Part model, mm, in its own coordinate system. Face numbers are marked on the shaded views. Give positions to 0.01 mm unless a question says otherwise; leave off trailing zeros. Loops run counter-clockwise (first coordinate to the right, second up) from the corner with the lowest first, then second, coordinate; pieces in that order, holes last. Notation, with made-up numbers: (53, 56) -> (85, 56) arc R15 ccw to (85, 60) -> close; hole circle Ø11 at (20, -1). An arc over 180 degrees is marked (long way). Write item = value, one per line.
from build123d import *

# Parameters (mm, degrees)
F3_R     = 3.8930000325
F4_DEPTH = 12.001


# Not quite as in the source:
# - a fillet or chamfer that OpenCascade refuses, or shapes differently, is made with other operations: its cross-section is extruded or revolved along the edge and cut away or added


with BuildPart() as f1:
    # F0 (on Front) → F1 (revolve)
    with BuildSketch(Plane.XZ):
        with BuildLine():
            Line((0, 12), (0, 0))
            Line((0, 0), (14.5, 0))
            ThreePointArc((14.5, 0), (14.8535533906, 0.1464466094), (15, 0.5))
            Line((15, 0.5), (15, 2))
            Line((15, 2), (5.4, 2))
            Line((5.4, 2), (4.6, 5))
            Line((4.6, 5), (4.6, 12))
            Line((4.6, 12), (0, 12))
        make_face()
    revolve(axis=Axis((0, 0, 6), (0, 0, 1)))

    # F3 (on face) → F4 (cut, through all)
    with BuildSketch(Plane.XY.offset(12)):
        Circle(F3_R)
    extrude(amount=-F4_DEPTH, mode=Mode.SUBTRACT)

    # F5: fillet of radius 1.5 on 1 edges, made by hand

    # F5_s1 → F5_t2 (revolve, cut)
    with BuildSketch(Plane.XZ):
        with BuildLine():
            ThreePointArc((3.8930000325, 12), (4.4113923991, 11.4549383915), (4.6, 10.7267557389))
            Line((4.6, 10.7267557389), (4.6, 12))
            Line((4.6, 12), (3.8930000325, 12))
        make_face()
    revolve(axis=Axis((0, 0, 12), (0, 0, 1)), mode=Mode.SUBTRACT)


solid = f1.part
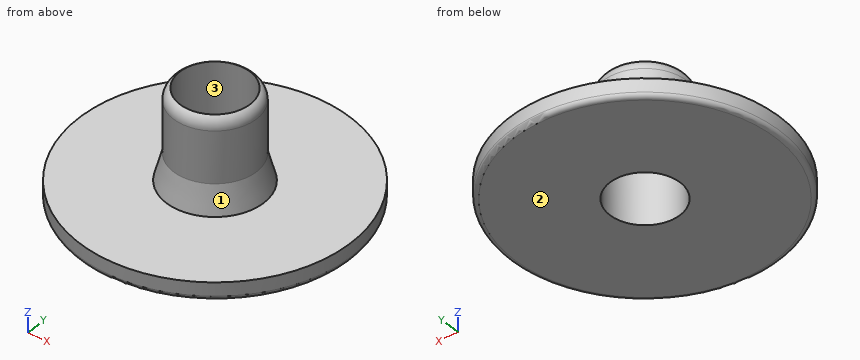
1) Pull direction X, two halves, no side cores. Call the marked faces 1, 2 and 3: pulls with the +X half, pulls with the -X half, needs draft (parallel to the pull), parting line crosses it, or undercut.
Resolved:
face_1 = parting line crosses it
face_2 = needs draft
face_3 = undercut
2) Slice it at D-D, the plane z = 1.25. List the corners of the cut face in (x, y), and give its area (3 significant figures).
Resolved:
outline = circle Ø30 at (0, 0); hole circle Ø7.79 at (0, 0)
area = 659 mm²
3) Slice it at C-C, the plane z = 4.25. List the corners of the cut face in (x, y), and give its area (3 significant figures).
Resolved:
outline = circle Ø9.6 at (0, 0); hole circle Ø7.79 at (0, 0)
area = 24.8 mm²
4) Slice it at A-A, the plane y = 0. List the corners of the cut face in (x, z).
Resolved:
outline = (-15, 0.5) arc R0.5 ccw to (-14.5, 0) -> (-3.89, 0) -> (-3.89, 12) arc R1.5 ccw to (-4.6, 10.73) -> (-4.6, 5) -> (-5.4, 2) -> (-15, 2) -> close; (3.89, 0) -> (14.5, 0) arc R0.5 ccw to (15, 0.5) -> (15, 2) -> (5.4, 2) -> (4.6, 5) -> (4.6, 10.73) arc R1.5 ccw to (3.89, 12) -> close
5) Drop flat-ended pins along their axis: P1, Ø4, axis at y = -3, z = 6, coming from the +X side; P2, Ø5, axis at x = 3, y = 7.5, coming from the +Z side; P3, Ø1.5, axis at x = -2.5, z = 8, coming from the -Y side. Give the stop position or say it passes through.
Resolved:
P1 = 4.49
P2 = 2
P3 = -4.25
6) Drill centre lines: line 1 along Y through (x, z) = (0, 7); line 2 along Z through (x, y) = (-6.5, 10); line 3 along Y through (x, z) = (2.5, 10.5). Where is each one in solid material? Low to high. Write a range as [from, to].
Resolved:
line_1 = [-4.6, -3.89], [3.89, 4.6]
line_2 = [0, 2]
line_3 = [-3.86, -2.98], [2.98, 3.86]
